Part model, mm, in its own coordinate system. A direction names the side the tool comes from. Coordinates: 2 decimals unless noted, no trailing zeros. Order: outer loops, then holes, each group sorted by start corner. A loop starts at its lowest first (then second) coordinate and runs counter-clockwise, first axis right, second up.
1) Tool access for faces 1 (the flat face through (0, -86.734, 7)), 2 (the flat face through (-6, 17, 0)), 3 (the cylindrical face through (0, -97, 3)), 4 (the flat face through (6, -97, 5)): list every direction of +Z, -Z, +X, -X, +Y, -Y with a clear straight run to the whole face (end or side of a thin tool).
2) Cut at C-C (y = -21.5). List the corners of the cut face in (x, z).
3) Cut at D-D (y = -4). List the corners of the cut face in (x, z), and give its area (3 significant figures).
4) Pin check, flat tips, straight feed: pin 1 Ø1.8 at (x, y) = (4.4, -99.73) entering from +Z; pin 2 Ø6.5 at (x, y) = (5, -93.5) entering from +Z; pin 3 Ø5 at (y, z) = (-98, 0.5) entering from -X; pin 4 Ø1.5 at (x, z) = (7, 7.5) entering from -Y. Stop position of each tip, or through.
5) Wall check: L1, parallel to Y at x = 12, z = 8.5; L2, parallel to Y at x = 0, z = -0.9; L3, parallel to X at y = 22, z = 0.25. Give the ranges that are in metal, low to high.
6) Mould opens along Y. For faces 5 (the flat face through (27.3, -25, 2)), 6 (the flat face through (0, -39, 5)), 7 (the flat face through (0, 34.766, 7)), 8 (the flat face through (0, -89.734, 4)) say: +Y half, -Y half, draft (parallel to the pull), parting line (faces both ways), or undercut.
7) Cut at B-B (z = 7.75). List the corners of the cut face in (x, y).
8) Cut at A-A (x = 0). List the corners of the cut face in (y, z), and give its area (3 significant figures).
Autodesk Inventor part; units mm, degrees
ref_plane "YZ Plane" through (0, 0, 0) normal (1, 0, 0) x (0, 1, 0)
ref_plane "XZ Plane" through (0, 0, 0) normal (0, 1, 0) x (-1, 0, 0)
ref_plane "XY Plane" through (0, 0, 0) normal (0, 0, 1) x (1, 0, 0)
sketch "Shutter" plane through (0, 0, 0) normal (0, 0, 1) x (1, 0, 0)
  line L0 (-25.5, 25.2655) -> (25.5, 25.2655)
  line L1 (25.5, 25.2655) -> (25.5, -25.7345)
  line L2 (25.5, -25.7345) -> (-25.5, -25.7345)
  line L3 (-25.5, -25.7345) -> (-25.5, 25.2655)
  line L4 (0, -25.7345) -> (0, 25.2655) construction
  circle A0 centre (0, -0.2345) radius 11 construction
  circle A1 centre (0, -0.2345) radius 17.5
  circle A2 centre (0, -0.2345) radius 20
  line L5 (-27.3, 37.7655) -> (-27.3, -89.7345)
  circle A3 centre (-4.3962, -99.7345) radius 1.5
  circle A4 centre (-4.3962, -94.7345) radius 1.5
  circle A5 centre (4.3962, -94.7345) radius 1.5
  circle A6 centre (4.3962, -99.7345) radius 1.5
  line L6 (27.3, 37.7655) -> (27.3, -89.7345)
  line L7 (-49, 0) -> (42, 0) construction
  line L8 (-27.3, 37.7655) -> (27.3, 37.7655)
  line L9 (-10, -104.7345) -> (10, -104.7345)
  line L10 (27.3, 37.7655) -> (-27.3, 37.7655)
  line L11 (-27.3, -89.7345) -> (27.3, -89.7345)
  line L12 (-27.3, -86.7345) -> (27.3, -86.7345)
  line L13 (0, -104.7345) -> (-10, -104.7345)
  line L14 (-10, -104.7345) -> (-10, -89.7345)
  line L15 (0, -104.7345) -> (10, -104.7345)
  line L16 (10, -104.7345) -> (10, -89.7345)
  point P0 (0, 17.2655)
  point P1 (0, 10.7655)
  dimension "d0" = 22
  dimension "d1" = 35
  dimension "d2" = 40
  dimension "d12" = 3
  dimension "d13" = 3
  dimension "d14" = 5
  dimension "d16" = 25.5
  dimension "d17" = 51
  dimension "d18" = 51
  dimension "d33" = 142.5
  dimension "d34" = 5
  dimension "d37" = 3
  dimension "d40" = 10
  dimension "d41" = 10
extrude "Extrusion1" add sketch "Shutter" against normal blind 1.5 contours L0 L1 L2 L3 | A2 | L8 L6 L12 L5 | L12 L6 L11 L5 | L11 L16 L9 L14
extrude "Extrusion2" add sketch "Shutter" along normal blind 5 contours L8 L6 L12 L5 | L12 L6 L11 L5 | L11 L16 L9 L14
ref_plane "Work Plane2" through (0, -85.7345, -1.5) normal (-1, 0, 0) x (0, 0, 1)
sketch "Sketch4" plane through (0, 0, 5) normal (0, 0, 1) x (1, 0, 0)
  line L0 (-27.3, 37.7655) -> (-27.3, -85.7345)
  line L1 (-27.3, 37.7655) -> (-27.3, 34.7655)
  line L2 (-27.3, 34.7655) -> (27.3, 34.7655)
  line L3 (27.3, -85.7345) -> (27.3, 37.7655)
  line L4 (27.3, 37.7655) -> (-27.3, 37.7655)
  line L5 (27.3, 37.7655) -> (-27.3, 37.7655)
  line L6 (-27.3, 34.7655) -> (-27.3, 37.7655)
  line L7 (27.3, 34.7655) -> (27.3, 37.7655)
  line L8 (27.3, -104.7345) -> (-10, -104.7345)
  line L9 (-27.3, -89.7345) -> (-27.3, 37.7655)
  line L10 (-27.3, -89.7345) -> (27.3, -89.7345)
  line L11 (27.3, 37.7655) -> (27.3, -89.7345)
  line L12 (27.3, -86.7345) -> (-27.3, -86.7345)
  line L13 (-27.3, -89.7345) -> (-27.3, -86.7345)
  line L14 (27.3, -89.7345) -> (27.3, -86.7345)
  point P0 (0, 0)
  dimension "d29" = 3
  dimension "d38" = 15
  dimension "d39" = 3
extrude "Extrusion4" add sketch "Sketch4" along normal blind 5 contours L4 L3 L2 L0 | L12 L11 L10 L9
sketch "Sketch5" plane through (-10, -104.7345, -1.5) normal (0, -1, 0) x (1, 0, 0)
  line L0 (0, 6.5) -> (20, 6.5)
  circle A0 centre (10, 6.5) radius 2
  dimension "d42" = 4
extrude "Extrusion5" cut sketch "Sketch5" against normal up to surface (15 mm away)
properties part number "PMT_Adaptor_Shutter"
Geometry check:
1. face 1: +Z, +X, -X
1. face 2: +Z
1. face 3: +Z, -Y
1. face 4: +Z, +X, -X, -Y
2. outline: (-27.3, -1.5) - (27.3, -1.5) - (27.3, 5) - (25.5, 5) - (25.5, 0) - (-25.5, 0) - (-25.5, 5) - (-27.3, 5) - close
3. outline: (-27.3, -1.5) - (-17.09, -1.5) - (-17.09, 0) - (-25.5, 0) - (-25.5, 5) - (-27.3, 5) - close; (17.09, -1.5) - (27.3, -1.5) - (27.3, 5) - (25.5, 5) - (25.5, 0) - (17.09, 0) - close
3. area: 48.6 mm2
4. pin 1: passes through
4. pin 2: stops at z = 5
4. pin 3: stops at x = -10
4. pin 4: stops at y = -89.73
5. L1: y = -89.73 to -86.73, 34.77 to 37.77
5. L2: y = -104.73 to -17.73, 17.27 to 37.77
5. L3: x = -27.3 to -25.5, 25.5 to 27.3
6. face 5: draft
6. face 6: undercut
6. face 7: undercut
6. face 8: -Y half
7. outline: (-27.3, -89.73) - (27.3, -89.73) - (27.3, -86.73) - (-27.3, -86.73) - close; (-27.3, 34.77) - (27.3, 34.77) - (27.3, 37.77) - (-27.3, 37.77) - close
8. outline: (-104.73, -1.5) - (-17.73, -1.5) - (-17.73, 0) - (-25.73, 0) - (-25.73, 5) - (-86.73, 5) - (-86.73, 10) - (-89.73, 10) - (-89.73, 3) - (-104.73, 3) - close; (17.27, -1.5) - (37.77, -1.5) - (37.77, 10) - (34.77, 10) - (34.77, 5) - (25.27, 5) - (25.27, 0) - (17.27, 0) - close
8. area: 619 mm2
